Geometry: final body of the model. Coordinates: model frame, mm. A direction names the side the tool comes from. Give positions to 0.01 mm unless a question says otherwise; leave off trailing zeros. Write each loop counter-clockwise with the first axis right and the second up, starting at its lowest first coordinate (ties: lowest second). Pieces come first, ordered by that corner, then holes. Notation, with made-up numbers: M 55,56 L 108,56 A33 cw 108,92 Z; hole C 52.5,-24.75 d8. An arc over 180 degrees is marked long. Use a Markdown table: item, result. Add a question column.
(1) Cut plane A-A (z = -2.5). Output: boundary loops of the cut face in (x, y).
(2) Material intervals for L1, parallel to X at y = 1.8, z = 3.5; L2, parallel to Y at x = 1.5, z = -2.5; L3, parallel to Z at x = 5.25, y = 0.5, sorted ascending.
(3) Draft query along Y for faces 4 (the flat face through (6, 1, 1)), 5 (the flat face through (0, 3, 3)), 6 (the cylindrical face through (-0.04, 1.45, -1.69)). Return one class per face: released by +Y, released by -Y, zero draft, split by the parting line, or undercut.
(4) Pin query (flat end, axial travel): pin 1 Ø1.2 at (x, y) = (-6, 1) entering from -Z; pin 2 Ø2.5 at (x, z) = (7.5, 3.5) entering from +Y; pin 3 Ø6 at (x, z) = (-5, 1.5) entering from +Y; pin 4 Ø1.5 at (x, y) = (3, 4.5) entering from +Z. Return the tip coordinate at first contact, or that it passes through.
(5) Cut plane D-D (z = 3.5). Output: boundary loops of the cut face in (x, y), plus the area to 4 significant figures.
(6) Cut plane C-C (x = 6.25). Output: boundary loops of the cut face in (y, z).
(7) Reachability of faces 1 (the cylindrical face through (0, 6.5, -2.6)), 2 (the flat face through (2.6, 1, -2)), 3 (the flat face through (-6, 1, 1)) from +Z, -Z, +X, -X, +Y, -Y: full face, straight path, thin tool, end or side. Return the list, or none.
(8) Cut plane B-B (y = 0.5). Output: boundary loops of the cut face in (x, z), plus the area to 3 significant figures.
```python
from build123d import *

# Parameters (mm, degrees)
SKIZZE1_W                       = 20
SKIZZE1_H                       = 12
AUFSATZ_LINEAR_AUSTRAGEN1_DEPTH = 3
SCHNITT_LINEAR_AUSTRAGEN1_REACH = 14.042
SKIZZE2_R                       = 1.5
AUFSATZ_LINEAR_AUSTRAGEN2_DEPTH = 20
FASE1_SIZE                      = 1.5
SKIZZE4_R                       = 1.75
SCHNITT_LINEAR_AUSTRAGEN2_DEPTH = 22.868927729
SKIZZE5_W                       = 7.4
SKIZZE5_H                       = 7
SCHNITT_LINEAR_AUSTRAGEN5_DEPTH = 14.351029923
FASE2_SIZE                      = 0.5
VERRUNDUNG1_R                   = 0.5
FASE3_SIZE                      = 0.5


with BuildPart() as part:
    # Skizze1 → Aufsatz-Linear austragen1 (new body)
    with BuildSketch(Plane(origin=(0, 0, 0), x_dir=(1, 0, 0), z_dir=(0, 1, 0))):
        Rectangle(SKIZZE1_W, SKIZZE1_H)
    extrude(amount=AUFSATZ_LINEAR_AUSTRAGEN1_DEPTH)

    # Skizze2 → Schnitt-Linear austragen1 (cut, up to next)
    with BuildSketch(Plane(origin=(0, 3, 0), x_dir=(1, 0, 0), z_dir=(0, 1, 0)), mode=Mode.PRIVATE) as schnitt_linear_austragen1_sk1:
        with Locations(Location((-7.5, -3.5, 0), (0, 0, 270))):
            Circle(SKIZZE2_R)
    schnitt_linear_austragen1_tool1 = extrude(schnitt_linear_austragen1_sk1.sketch, amount=-SCHNITT_LINEAR_AUSTRAGEN1_REACH, mode=Mode.PRIVATE) & part.part
    # Skizze2 → Schnitt-Linear austragen1 (cut, up to next)
    with BuildSketch(Plane(origin=(0, 3, 0), x_dir=(1, 0, 0), z_dir=(0, 1, 0)), mode=Mode.PRIVATE) as schnitt_linear_austragen1_sk2:
        with Locations(Location((7.5, -3.5, 0), (0, 0, 270))):
            Circle(SKIZZE2_R)
    schnitt_linear_austragen1_tool2 = extrude(schnitt_linear_austragen1_sk2.sketch, amount=-SCHNITT_LINEAR_AUSTRAGEN1_REACH, mode=Mode.PRIVATE) & part.part
    add(schnitt_linear_austragen1_tool1.solids().sort_by_distance((-7.5, 3, 3.5))[0], mode=Mode.SUBTRACT)
    add(schnitt_linear_austragen1_tool2.solids().sort_by_distance((7.5, 3, 3.5))[0], mode=Mode.SUBTRACT)

    # Skizze3 → Aufsatz-Linear austragen2 (add)
    with BuildSketch(Plane.ZY.offset(10)):
        with BuildLine():
            Line((-6, 3), (1, 3))
            ThreePointArc((1, 3), (-2.5, 6.5), (-6, 3))
        make_face()
    extrude(amount=-AUFSATZ_LINEAR_AUSTRAGEN2_DEPTH)

    # Fase1
    fase1_edges = [part.edges().sort_by_distance(p)[0] for p in [
        (10, 1.5, 6),
        (-10, 1.5, 6),
    ]]
    chamfer(fase1_edges, length=FASE1_SIZE)

    # Skizze4 → Schnitt-Linear austragen2 (cut, through all)
    with BuildSketch(Plane.ZY.offset(10)):
        with Locations((-2.5, 3)):
            Circle(SKIZZE4_R)
    extrude(amount=-SCHNITT_LINEAR_AUSTRAGEN2_DEPTH, mode=Mode.SUBTRACT)

    # Skizze5 → Schnitt-Linear austragen5 (cut, through all)
    with BuildSketch(Plane(origin=(0, 0, 0), x_dir=(1, 0, 0), z_dir=(0, 1, 0))):
        with Locations((-6.3, 2.5)):
            Rectangle(SKIZZE5_W, SKIZZE5_H)
        with Locations((6.3, 2.5)):
            Rectangle(SKIZZE5_W, SKIZZE5_H)
    extrude(amount=SCHNITT_LINEAR_AUSTRAGEN5_DEPTH, mode=Mode.SUBTRACT)

    # Fase2
    fase2_edges = [part.edges().sort_by_distance(p)[0] for p in [
        (-10, 3, 2.75),
        (6.3, 3, 1),
        (10, 3, 2.75),
        (0, 3, 6),
        (-9.25, 3, 5.25),
        (9.25, 3, 5.25),
        (-6.3, 3, 1),
    ]]
    chamfer(fase2_edges, length=FASE2_SIZE)

    # Verrundung1
    verrundung1_edges = [part.edges().sort_by_distance(p)[0] for p in [
        (0, 3, 1),
    ]]
    fillet(verrundung1_edges, radius=VERRUNDUNG1_R)

    # Fase3
    # the kernel refuses this chamfer: 0.5 mm, written as the material it takes off along each edge
    with BuildSketch(Plane(origin=(2.6, 3, 1.468626967), x_dir=(-0.9996219169112968, 0.027495876610586487, 0), z_dir=(0, 0, 1))) as fase3_piece_1_section:
        Polygon((FASE3_SIZE * 0.999621916911, FASE3_SIZE * 0.0274958766106), (-FASE3_SIZE * 0.0274958766106, FASE3_SIZE * 0.999621916911), (0, 0), align=None)
    fase3_piece_1 = extrude(amount=1.317214527, mode=Mode.PRIVATE)
    fase3_piece_1 = split(fase3_piece_1, bisect_by=Plane(origin=(2.355172989, 2.984397258, 1.484397258), z_dir=(0, 0.7071067811865476, -0.7071067811865476)), keep=Keep.TOP, mode=Mode.PRIVATE)
    add(fase3_piece_1, mode=Mode.SUBTRACT)
    with BuildSketch(Plane(origin=(-2.6, 3, 1.468626967), x_dir=(0.9996219169112968, 0.027495876610586487, 0), z_dir=(0, 0, 1))) as fase3_piece_2_section:
        Polygon((FASE3_SIZE * 0.999621916911, -FASE3_SIZE * 0.0274958766106), (-FASE3_SIZE * 0.0274958766106, -FASE3_SIZE * 0.999621916911), (0, 0), align=None)
    fase3_piece_2 = extrude(amount=1.317214527, mode=Mode.PRIVATE)
    fase3_piece_2 = split(fase3_piece_2, bisect_by=Plane(origin=(-2.355172989, 2.984397258, 1.484397258), z_dir=(0, 0.7071067811865476, -0.7071067811865476)), keep=Keep.TOP, mode=Mode.PRIVATE)
    add(fase3_piece_2, mode=Mode.SUBTRACT)
    with BuildSketch(Plane(origin=(2.6, 3, -2.5), x_dir=(0, 0.125, 0.9921567416492215), z_dir=(0, -0.9921567416492215, 0.125))) as fase3_piece_3:
        Polygon((3.5 - FASE3_SIZE, 0), (3.5, FASE3_SIZE), (3.5, 0), align=None)
    revolve(axis=Axis((2.6, 3, -2.5), (-1, 0, 0)), revolution_arc=172.819244219, mode=Mode.SUBTRACT)
    with BuildSketch(Plane(origin=(-2.6, 3.5, 1.468626967), x_dir=(0, -1, 0), z_dir=(0, 0, 1))) as fase3_piece_4_section:
        Polygon((0.5, FASE3_SIZE), (0.5 + FASE3_SIZE, 0), (0.5, 0), align=None)
    fase3_piece_4 = revolve(axis=Axis((-2.6, 3.5, 1.468626967), (1, 0, 0)), revolution_arc=82.819244219, mode=Mode.PRIVATE)
    fase3_piece_4 = split(fase3_piece_4, bisect_by=Plane(origin=(-2.375928001, 2.853387765, 1.353387765), z_dir=(0, 0.7071067811865476, -0.7071067811865476)), keep=Keep.TOP, mode=Mode.PRIVATE)
    add(fase3_piece_4, mode=Mode.SUBTRACT)
    with BuildSketch(Plane(origin=(2.6, 3.5, 1.468626967), x_dir=(0, -1, 0), z_dir=(0, 0, 1))) as fase3_piece_5_section:
        Polygon((0.5 + FASE3_SIZE, 0), (0.5, -FASE3_SIZE), (0.5, 0), align=None)
    fase3_piece_5 = revolve(axis=Axis((2.6, 3.5, 1.468626967), (1, 0, 0)), revolution_arc=82.819244219, mode=Mode.PRIVATE)
    fase3_piece_5 = split(fase3_piece_5, bisect_by=Plane(origin=(2.437201985, 2.797231412, 1.297231412), z_dir=(0, 0.7071067811865476, -0.7071067811865476)), keep=Keep.TOP, mode=Mode.PRIVATE)
    add(fase3_piece_5, mode=Mode.SUBTRACT)
    with BuildSketch(Plane(origin=(-2.6, 3, -2.5), x_dir=(0, 0.125, 0.9921567416492215), z_dir=(0, -0.9921567416492215, 0.125))) as fase3_piece_6:
        Polygon((3.5 - FASE3_SIZE, 0), (3.5, -FASE3_SIZE), (3.5, 0), align=None)
    revolve(axis=Axis((-2.6, 3, -2.5), (-1, 0, 0)), revolution_arc=172.819244219, mode=Mode.SUBTRACT)
    with BuildSketch(Plane(origin=(-2.6, -1.285841494, -6), x_dir=(-0.02749587661058651, 0, 0.9996219169112968), z_dir=(0, 1, 0))) as fase3_piece_7:
        Polygon((FASE3_SIZE * 0.999621916911, FASE3_SIZE * 0.0274958766106), (-FASE3_SIZE * 0.0274958766106, FASE3_SIZE * 0.999621916911), (0, 0), align=None)
    extrude(amount=4.285841494, mode=Mode.SUBTRACT)
    with BuildSketch(Plane(origin=(2.6, -1.285841494, -6), x_dir=(0.02749587661058651, 0, 0.9996219169112968), z_dir=(0, 1, 0))) as fase3_piece_8:
        Polygon((FASE3_SIZE * 0.999621916911, -FASE3_SIZE * 0.0274958766106), (-FASE3_SIZE * 0.0274958766106, -FASE3_SIZE * 0.999621916911), (0, 0), align=None)
    extrude(amount=4.285841494, mode=Mode.SUBTRACT)


solid = part.part
```
Answer list:
| question | item | result |
|---|---|---|
| 1 | outline | M -2.6,0 L 2.6,0 L 2.6,1.25 L -2.6,1.25 Z; M -2.6,4.75 L 2.6,4.75 L 2.6,6 L 2.1,6.5 L -2.1,6.5 L -2.6,6 Z |
| 2 | L1 | -10 to -9, -6 to 6, 9 to 10 |
| 2 | L2 | 0 to 1.25, 4.75 to 6.5 |
| 2 | L3 | 1 to 6 |
| 3 | face 4 | zero draft |
| 3 | face 5 | released by +Y |
| 3 | face 6 | undercut |
| 4 | pin 1 | z = 1 |
| 4 | pin 2 | through |
| 4 | pin 3 | y = 5.04 |
| 4 | pin 4 | z = 0.56 |
| 5 | outline | M -10,0 L -9,0 L -9,3 L -9.5,3 L -10,2.5 Z; M -6,0 L 6,0 L 6,3 L -6,3 Z; M 9,0 L 10,0 L 10,2.5 L 9.5,3 L 9,3 Z |
| 5 | area | 41.75 mm² |
| 6 | outline | M 0,1 L 2.5,1 L 3,1.5 L 3,2.67 L 0,2.67 Z; M 0,4.33 L 3,4.33 L 3,5.5 L 2.5,6 L 0,6 Z |
| 7 | face 1 | +X, -X, +Y |
| 7 | face 2 | -Z, +X, +Y, -Y |
| 7 | face 3 | -Z, -X, +Y, -Y |
| 8 | outline | M -10,1 L -2.6,1 L -2.6,-5.5 L -2.1,-6 L 2.1,-6 L 2.6,-5.5 L 2.6,1 L 10,1 L 10,4.5 L 8.5,6 L -8.5,6 L -10,4.5 Z; hole C -7.5,3.5 d3; hole C 7.5,3.5 d3 |
| 8 | area | 120 mm² |
